Autodesk Fusion 360 part; units mm, degrees
sketch "pik-sk" plane through (0, 0, 0) normal (0, 0, 1) x (1, 0, 0)
  line L0 (-49.6541, 34.7973) -> (-49.6541, 23.1738)
  line L1 (-49.6541, 23.1738) -> (-45.9923, 23.1738)
  line L2 (-45.9923, 23.1738) -> (-45.9923, 17.5515)
  line L3 (-45.9923, 17.5515) -> (-42.3651, 17.5515)
  line L4 (-42.3651, 17.5515) -> (-42.3651, 11.6579)
  line L5 (-42.3651, 11.6579) -> (-38.829, 11.6579)
  line L6 (-38.829, 11.6579) -> (-38.829, 8.6694)
  line L7 (-38.829, 8.6694) -> (-35.4308, 8.6694)
  line L8 (-35.4308, 8.6694) -> (-35.4308, 5.7405)
  line L9 (-35.4308, 5.7405) -> (-32.068, 5.7405)
  line L10 (-32.068, 5.7405) -> (-32.068, 0.0385)
  line L11 (-32.068, 0.0385) -> (-35.4308, 0.0385)
  line L12 (-35.4308, 0.0385) -> (-35.4308, -11.6953)
  line L13 (-35.4308, -11.6953) -> (-38.9575, -11.6953)
  line L14 (-38.9575, -11.6953) -> (-38.9575, -20.569)
  line L15 (-38.9575, -20.569) -> (-35.4308, -20.569)
  line L16 (-35.4308, -20.569) -> (-35.4308, -23.2957)
  line L17 (-35.4308, -23.2957) -> (-32.0468, -23.2957)
  line L18 (-32.0468, -23.2957) -> (-32.0468, -26.1695)
  line L19 (-32.0468, -26.1695) -> (-28.3803, -26.1695)
  line L20 (-28.3803, -26.1695) -> (-28.3803, -29.3405)
  line L21 (-28.3803, -29.3405) -> (-21.2455, -29.3405)
  line L22 (-21.2455, -29.3405) -> (-21.2455, -32.1152)
  line L23 (-21.2455, -32.1152) -> (-10.7414, -32.1152)
  line L24 (-10.7414, -32.1152) -> (-10.7414, -34.8898)
  line L25 (-10.7414, -34.8898) -> (0.0599, -34.8898)
  line L26 (0, 14.6559) -> (-6.8686, 14.6476)
  line L27 (-6.8686, 14.6476) -> (-6.8721, 17.5432)
  line L28 (-6.8721, 17.5432) -> (-13.9652, 17.5346)
  line L29 (-13.9652, 17.5346) -> (-13.9687, 20.3821)
  line L30 (-13.9687, 20.3821) -> (-21.0302, 20.3735)
  line L31 (-21.0302, 20.3735) -> (-21.0339, 23.4685)
  line L32 (-21.0339, 23.4685) -> (-24.6974, 23.4641)
  line L33 (-24.6974, 23.4641) -> (-24.7009, 26.3367)
  line L34 (-24.7009, 26.3367) -> (-31.8504, 26.3281)
  line L35 (-31.8504, 26.3281) -> (-31.8539, 29.2052)
  line L36 (-31.8539, 29.2052) -> (-35.372, 29.2009)
  line L37 (-35.372, 29.2009) -> (-35.3755, 32.1099)
  line L38 (-35.3755, 32.1099) -> (-42.492, 32.1013)
  line L39 (-42.492, 32.1013) -> (-42.4954, 34.8818)
  line L40 (-42.4954, 34.8818) -> (-49.6541, 34.8818)
  line L41 (-49.6541, 34.8818) -> (-49.6541, 34.7973)
  line L42 (32.0895, 5.8181) -> (32.1032, 0.1161)
  line L43 (35.4451, 8.7551) -> (35.4522, 5.8262)
  line L44 (42.358, 17.6539) -> (42.3722, 11.7604)
  line L45 (31.8186, 29.2822) -> (35.3367, 29.2864)
  line L46 (42.4463, 34.9845) -> (49.605, 35.0018)
  line L47 (21.0163, 20.4244) -> (21.0125, 23.5194)
  line L48 (31.8221, 26.4051) -> (31.8186, 29.2822)
  line L49 (24.6761, 23.5238) -> (24.6726, 26.3964)
  line L50 (42.4497, 32.2039) -> (42.4463, 34.9845)
  line L51 (6.8651, 17.5598) -> (13.9582, 17.5684)
  line L52 (13.9548, 20.4158) -> (21.0163, 20.4244)
  line L53 (0, 14.6559) -> (6.8686, 14.6642)
  line L54 (32.1454, -26.0919) -> (28.4789, -26.1007)
  line L55 (21.3518, -29.289) -> (21.3585, -32.0637)
  line L56 (35.5224, -23.21) -> (32.1385, -23.2181)
  line L57 (35.4944, -11.6095) -> (39.0211, -11.601)
  line L58 (6.8686, 14.6642) -> (6.8651, 17.5598)
  line L59 (35.4522, 5.8262) -> (32.0895, 5.8181)
  line L60 (21.0125, 23.5194) -> (24.6761, 23.5238)
  line L61 (35.3332, 32.1953) -> (42.4497, 32.2039)
  line L62 (42.3722, 11.7604) -> (38.8361, 11.7518)
  line L63 (45.9852, 17.6627) -> (42.358, 17.6539)
  line L64 (49.6052, 34.9173) -> (49.6334, 23.2938)
  line L65 (24.6726, 26.3964) -> (31.8221, 26.4051)
  line L66 (32.1032, 0.1161) -> (35.466, 0.1242)
  line L67 (28.4866, -29.2718) -> (21.3518, -29.289)
  line L68 (35.466, 0.1242) -> (35.4944, -11.6095)
  line L69 (38.8361, 11.7518) -> (38.8433, 8.7633)
  line L70 (38.8433, 8.7633) -> (35.4451, 8.7551)
  line L71 (10.8545, -32.0891) -> (10.8612, -34.8637)
  line L72 (49.605, 35.0018) -> (49.6052, 34.9173)
  line L73 (10.8612, -34.8637) -> (0.0599, -34.8898)
  line L74 (49.6334, 23.2938) -> (45.9716, 23.2849)
  line L75 (32.1385, -23.2181) -> (32.1454, -26.0919)
  line L76 (39.0211, -11.601) -> (39.0425, -20.4747)
  line L77 (35.5158, -20.4832) -> (35.5224, -23.21)
  line L78 (39.0425, -20.4747) -> (35.5158, -20.4832)
  line L79 (35.3367, 29.2864) -> (35.3332, 32.1953)
  line L80 (45.9716, 23.2849) -> (45.9852, 17.6627)
  line L81 (13.9582, 17.5684) -> (13.9548, 20.4158)
  line L82 (28.4789, -26.1007) -> (28.4866, -29.2718)
  line L83 (21.3585, -32.0637) -> (10.8545, -32.0891)
extrude "Extrude1" add sketch "pik-sk" along normal blind 10
Read the model definition and answer for the solid it produces. Units are mm, in the model's axes. A direction names the side the tool comes from. Coordinates: 2 decimals unless noted, no trailing zeros. Loops run counter-clockwise (first coordinate to the right, second up) from the corner with the lowest first, then second, coordinate; pieces in that order, holes last. Notation, with made-up numbers: (39, 19) -> (86, 19) arc R24 cw to (86, 47) -> close; hole circle Ø2 at (62.5, 43). An arc over 180 degrees is marked (long way). Return JSON: item names as keys, results as strings.
Item 1: For faces 1 (the flat face through (-16, -32.115, 5)), 2 (the flat face through (-37, 8.669, 5)), 3 (the flat face through (-5, -34.89, 5)), determine the directions among +Z, -Z, +X, -X, +Y, -Y from which every point of the face is accessible in a straight line to the end or side of a thin tool.
Answers:
{"face 1": "+Z, -Z, -X, -Y", "face 2": "+Z, -Z, -X", "face 3": "+Z, -Z, +X, -X, -Y"}
Item 2: Flat-ended cylindrical pins translate along their axes: P1, Ø2, axis at x = 1.5, z = 6, coming from the -Y side; P2, Ø3.5, axis at x = -34.5, z = 6, coming from the -Y side; P3, Ø3, axis at y = 10, z = 3, coming from the -X side; P4, Ø2, axis at y = -11.5, z = 6.5, coming from the -X side. Find the tip coordinate at first contact, or state that the pin passes through.
Answers:
{"P1": "stops at y = -34.89", "P2": "stops at y = -23.3", "P3": "stops at x = -38.83", "P4": "stops at x = -38.96"}
Item 3: Find section C-C (x = -26.5). Determine the outline of the cut face in (y, z).
Answers:
{"outline": "(-29.34, 0) -> (26.33, 0) -> (26.33, 10) -> (-29.34, 10) -> close"}
Item 4: Find section D-D (y = -7.5). Determine the outline of the cut face in (x, z), plus the area to 3 significant figures.
Answers:
{"outline": "(-35.43, 0) -> (35.48, 0) -> (35.48, 10) -> (-35.43, 10) -> close", "area": "709 mm2"}
Item 5: Find the intervals of material crossed by probe 1 along X at (y, z) = (27, 8.5); probe 2 along Y at (x, z) = (37.5, 1); probe 3 along X at (y, z) = (20.5, 9.5), in increasing order.
Answers:
{"probe 1": "x = -49.65 to -31.85, 31.82 to 49.62", "probe 2": "y = -20.48 to -11.6, 8.76 to 32.2", "probe 3": "x = -45.99 to -21.03, 21.02 to 45.98"}
Item 6: Find section A-A (x = 34). Determine the outline of the cut face in (y, z).
Answers:
{"outline": "(-23.21, 0) -> (0.12, 0) -> (0.12, 10) -> (-23.21, 10) -> close; (5.82, 0) -> (29.28, 0) -> (29.28, 10) -> (5.82, 10) -> close"}
Item 7: Find section B-B (y = 27.5). Determine the outline of the cut face in (x, z), plus the area to 3 significant figures.
Answers:
{"outline": "(-49.65, 0) -> (-31.85, 0) -> (-31.85, 10) -> (-49.65, 10) -> close; (31.82, 0) -> (49.62, 0) -> (49.62, 10) -> (31.82, 10) -> close", "area": "356 mm2"}
